The listing builds one solid part. Answer for the finished solid, in the listing's coordinates (mm). Face numbers are marked on the shaded views. A direction names the side the tool comes from. Coordinates: 2 decimals unless noted, no trailing zeros. Loops run counter-clockwise (first coordinate to the right, second up) from the corner with the lowest first, then second, coordinate; pieces in that order, holes last. Notation, with made-up numbers: (83, 60.5) - (113, 60.5) arc R19 ccw to (113, 91.5) - close; hole circle Ø3 at (88.5, 59.5). An arc over 180 degrees is marked (long way). One line per question, with ' | ' between items.
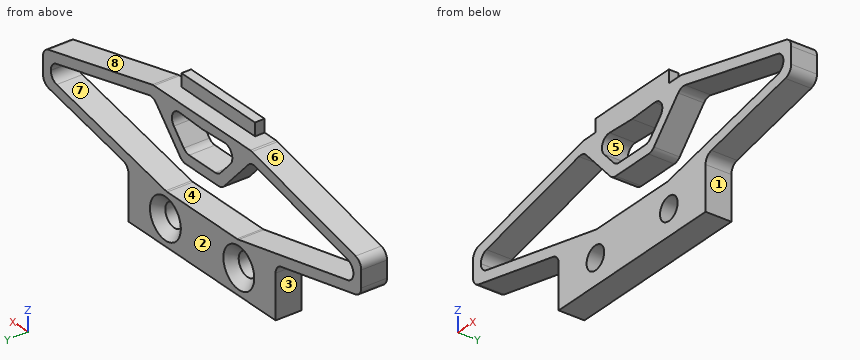
from build123d import *

# Parameters (mm, degrees)
BOSS_EXTRUDE1_DEPTH                                 = 4
FILLET1_R                                           = 1.5
CSK_FOR_M3_COUNTERSUNK_FLAT_HEAD_SCREW1_D           = 3.6
CSK_FOR_M3_COUNTERSUNK_FLAT_HEAD_SCREW1_CSINK_D     = 6.3
CSK_FOR_M3_COUNTERSUNK_FLAT_HEAD_SCREW1_CSINK_ANGLE = 90
SKETCH5_W                                           = 7.5
SKETCH5_H                                           = 1.5
BOSS_EXTRUDE2_DEPTH                                 = 2


with BuildPart() as part:
    # Sketch1 → Boss-Extrude1 (new body)
    with BuildSketch(Plane(origin=(0, 0, 0), x_dir=(1, 0, 0), z_dir=(0, 1, 0))):
        Polygon((0, 0), (-15, 0), (-15, -8), (-32.5, -11.703142934), (-32.5, -16.703142934), (-10, -22), (0, -22), (0, -20.4), (-8.217014563, -20.776004397), (-3.311485397, -15.4), (0, -15.4), (0, -13.8), (-4.017502815, -13.8), (-10, -20.356261329), (-30.9, -15.436069655), (-30.9, -13), (-7.271422452, -8), (0, -8), align=None)
    extrude(amount=BOSS_EXTRUDE1_DEPTH)

    # Fillet1
    fillet1_edges = [part.edges().sort_by_distance(p)[0] for p in [
        (-7.271422452, 2, 8),
        (-30.9, 2, 13),
        (-30.9, 2, 15.436069655),
        (-10, 2, 20.356261329),
        (-4.017502815, 2, 13.8),
        (-3.311485397, 2, 15.4),
        (-8.217014563, 2, 20.776004397),
        (-10, 2, 22),
        (-32.5, 2, 16.703142934),
        (-32.5, 2, 11.703142934),
        (-15, 2, 8),
    ]]
    fillet(fillet1_edges, radius=FILLET1_R)

    # CSK for M3 Countersunk Flat Head Screw1 (through all)
    with Locations(Plane(origin=(0, 4, 0), x_dir=(1, 0, 0), z_dir=(0, 1, 0))):
        with Locations((-7.5, -4)):
            CounterSinkHole(CSK_FOR_M3_COUNTERSUNK_FLAT_HEAD_SCREW1_D / 2, CSK_FOR_M3_COUNTERSUNK_FLAT_HEAD_SCREW1_CSINK_D / 2, counter_sink_angle=CSK_FOR_M3_COUNTERSUNK_FLAT_HEAD_SCREW1_CSINK_ANGLE)

    # Sketch5 → Boss-Extrude2 (add)
    with BuildSketch(Plane.XY.offset(22)):
        with Locations((-3.75, 0.75)):
            Rectangle(SKETCH5_W, SKETCH5_H)
    extrude(amount=BOSS_EXTRUDE2_DEPTH)

    # Mirror1: part across plane


with BuildPart() as part_1:
    add(part.part)
    add(part.part.mirror(Plane(origin=(0, 4, 8), x_dir=(0, 0, 1), z_dir=(-1, 0, 0))))


solid = part_1.part
Item 1: Find section C-C, the plane y = 3.25. State how many separate pieces and enclosed holes the cut face has, plus the area to 3 significant figures.
Taken from the geometry:
separate pieces: 1 | enclosed holes: 4 | area: 427 mm2
Item 2: Find section D-D, the plane x = 13.5. Write down the section's boundary in (y, z), plus the area to 3 significant figures.
Taken from the geometry:
outline: (0, 0) - (4, 0) - (4, 9.32) - (0, 9.32) - close; (0, 19.53) - (4, 19.53) - (4, 21.18) - (0, 21.18) - close | area: 43.8 mm2
Item 3: Find section A-A, the plane z = 4. Write down the section's boundary in (x, y), plus the area to 3 significant figures.
Taken from the geometry:
outline: (-15, 0) - (-9.3, 0) - (-9.3, 2.65) - (-10.65, 4) - (-15, 4) - close; (-5.7, 0) - (5.7, 0) - (5.7, 2.65) - (4.35, 4) - (-4.35, 4) - (-5.7, 2.65) - close; (9.3, 0) - (15, 0) - (15, 4) - (10.65, 4) - (9.3, 2.65) - close | area: 87.6 mm2
Item 4: Each of these flat-tipped pins is pushed along its axis until it touches: pin 1 Ø2 at (y, z) = (1.5, 2) entering from -X; pin 2 Ø2 at (x, y) = (1, 1.5) entering from -Z; pin 3 Ø2 at (y, z) = (3, 17) entering from -X; pin 4 Ø1.2 at (y, z) = (1, 23) entering from -X. Where does it stop, or does it pass through?
Taken from the geometry:
pin 1: stops at x = -15 | pin 2: stops at z = 0 | pin 3: stops at x = -32.42 | pin 4: stops at x = -7.5
Item 5: Find section B-B, the plane x = -28. Write down the section's boundary in (y, z).
Taken from the geometry:
outline: (0, 10.75) - (4, 10.75) - (4, 12.39) - (0, 12.39) - close; (0, 16.12) - (4, 16.12) - (4, 17.76) - (0, 17.76) - close
Item 6: Which of the six approach directions +Z, -Z, +X, -X, +Y, -Y give full straight-line access (tool end or side, diameter ignored) to the marked faces 1, 2, 3 and 4?
Taken from the geometry:
face 1: -Z, +X, +Y, -Y | face 2: +Z, -Z, +X, -X, +Y | face 3: -Z, -X, +Y, -Y | face 4: +Y, -Y
Item 7: Find the intervals of material crossed by line 1 (X direction, y = 1.25, z = 4); line 2 (Z direction, x = 7.5, y = 1.8); line 3 (Z direction, x = 4, y = 3.7), in increasing order. Write a range as [from, to].
Taken from the geometry:
line 1: x = [-15, -9.3], [-5.7, 5.7], [9.3, 15] | line 2: z = [0, 2.2], [5.8, 8.05], [17.62, 22] | line 3: z = [0, 8], [13.95, 16.15], [20.58, 22]
Item 8: The mould has two halves that part along X. Classify the marked faces 5, 6, 7 and 8: pulls with the +X half, pulls with the -X half, needs draft (parallel to the pull), parting line crosses it, or undercut.
Taken from the geometry:
face 5: undercut | face 6: pulls with the -X half | face 7: undercut | face 8: pulls with the +X half
